```python
from build123d import *

# Parameters (mm, degrees)
F1_DEPTH = 25


# Not quite as in the source:
# - ends of sketch curves that miss each other by under 0.0002 mm in the source are joined


with BuildPart() as f1:
    # F0 (on Front) → F1 (new body)
    with BuildSketch(Plane.XZ):
        Polygon((-275, 53.7867965644), (-275, -275), (275, -275), (275, 275), (-68.7867965644, 275), (-68.7867965644, 260), (115, 260), (115, 267.5000010639), (130, 267.5000010639), (130, 260), (260, 260), (260, -35), (267.5, -35), (267.5, -50), (260, -50), (260, -260), (50, -260), (50, -267.5), (35, -267.5), (35, -260), (-260, -260), (-260, -130), (-267.5, -130), (-267.5, -115), (-260, -115), (-260, 68.7867965644), (-268.7268512791, 60.0599452853), align=None)
        Polygon((-275, 68.7867965644), (-275, 53.7867965644), (-268.7268512791, 60.0599452853), (-260, 68.7867965644), align=None)
        Polygon((-275, 75), (-275, 68.7867965644), (-260, 68.7867965644), align=None)
        Polygon((-68.7867965644, 260), (-68.7867965644, 275), (-75, 275), align=None)
        Polygon((-79.3933982822, 270.6066017178), (-275, 75), (-260, 68.7867965644), (-68.7867965644, 260), align=None)
        Polygon((-68.7867965644, 260), (-75, 275), (-79.3933982822, 270.6066017178), align=None)
        Polygon((-260, -122.5), (-260, -115), (-267.5, -115), (-267.5, -130), (-260, -130), (35, -130), (35, -260), (35, -267.5), (50, -267.5), (50, -260), (50, -115), (42.5, -115), (42.5, -122.5), (41.5, -122.5), (41.5, -115), (39.3933982822, -115), (-44.3324317381, -115), (-45, -115), (-45, -122.5), (-46, -122.5), (-46, -115), (-258.5857843554, -115), (-259, -115), (-259, -115.414213564), (-259, -122.5), align=None)
        Polygon((115, 267.5000010639), (115, 260), (122.5, 260), (122.5, 259), (115.414213564, 259), (115, 259), (115, 258.5857864337), (115, 46), (122.5, 46), (122.5, 45), (115, 45), (115, -41.5), (122.5, -41.5), (122.5, -42.5), (115, -42.5), (115, -50), (260, -50), (267.5, -50), (267.5, -35), (260, -35), (130, -35), (130, 260), (130, 267.5000010639), align=None)
    extrude(amount=F1_DEPTH)


solid = f1.part
```
The model under review builds one solid part; all positions refer to its coordinate system, in mm. A direction names the side the tool comes from. Give positions to 0.01 mm unless a question says otherwise; leave off trailing zeros. Write each loop counter-clockwise with the first axis right and the second up, starting at its lowest first coordinate (ties: lowest second). Pieces come first, ordered by that corner, then holes. Notation, with made-up numbers: M 18,46 L 66,46 A20 ccw 66,65 Z; hole C 16.25,35.5 d8. An arc over 180 degrees is marked long. Answer in a Markdown table with one row per item.
Item 1: For line 1 along X through (y, z) = (-7.25, 52); line 2 along Z through (x, y) = (206, -24); line 3 along Z through (x, y) = (-24.5, -6.75), list the stretches that pass through material, from the lowest coordinate up.
Check sheet entries:
| item | result |
|---|---|
| line 1 | -275 to -260, 115 to 130, 260 to 275 |
| line 2 | -275 to -260, -50 to -35, 260 to 275 |
| line 3 | -275 to -260, -130 to -115, 260 to 275 |
Item 2: Add section B-B on x = 169. Give the boundary of the cut face in (y, z).
Check sheet entries:
| item | result |
|---|---|
| outline | M -25,-275 L 0,-275 L 0,-260 L -25,-260 Z; M -25,-50 L 0,-50 L 0,-35 L -25,-35 Z; M -25,260 L 0,260 L 0,275 L -25,275 Z |
Item 3: Draft analysis for pull direction X (two halves, no side actions). For faces 1 (the face through (275, -12, -4)), 2 (the face through (-275, -12, -98)), 3 (the face through (-4, -12, -275)), 4 (the face through (-151, -12, -115)), state which applies: +X half, -X half, draft (parallel to the pull), parting line (faces both ways), or undercut.
Check sheet entries:
| item | result |
|---|---|
| face 1 | +X half |
| face 2 | -X half |
| face 3 | draft |
| face 4 | undercut |
Item 4: Tool access review of faces 5 (the face through (121, -25, -19)), 6 (the face through (156, -12, -260)): name each direction out of +Z, -Z, +X, -X, +Y, -Y from which nothing blocks a thin tool from reaching the whole face with its end or side.
Check sheet entries:
| item | result |
|---|---|
| face 5 | +Z, -Z, +X, -X, -Y |
| face 6 | +Y, -Y |
Item 5: Add section A-A on z = -138. Give the boundary of the cut face in (x, y), plus the area to 4 significant figures.
Check sheet entries:
| item | result |
|---|---|
| outline | M -275,-25 L -260,-25 L -260,0 L -275,0 Z; M 35,-25 L 50,-25 L 50,0 L 35,0 Z; M 260,-25 L 275,-25 L 275,0 L 260,0 Z |
| area | 1,125 mm2 |
Item 6: Add section C-C on z = -63. Give the boundary of the cut face in (x, y).
Check sheet entries:
| item | result |
|---|---|
| outline | M -275,-25 L -260,-25 L -260,0 L -275,0 Z; M 260,-25 L 275,-25 L 275,0 L 260,0 Z |
Item 7: For P1, Ø1.1, axis at y = -12.5, z = 259.5, coming from the -X side; P2, Ø7.5, axis at x = -180, y = -6.5, coming from the +Z side, all flat-tipped, find the tip position at first contact; note any pin that passes through.
Check sheet entries:
| item | result |
|---|---|
| P1 | x = -91.05 |
| P2 | z = 173.75 |
Item 8: Add section D-D on x = 102. Give the boundary of the cut face in (y, z).
Check sheet entries:
| item | result |
|---|---|
| outline | M -25,-275 L 0,-275 L 0,-260 L -25,-260 Z; M -25,260 L 0,260 L 0,275 L -25,275 Z |
